```python
from build123d import *

# Parameters (mm, degrees)
BOSS_EXTRUDE2_START      = 6
BOSS_EXTRUDE2_DEPTH      = 44
SKETCH2_R                = 16.25
CUT_EXTRUDE1_DEPTH       = 1
CUT_EXTRUDE1_DEPTH_BACK  = 45
CUT_EXTRUDE3_DEPTH       = 45
FILLET1_R                = 3
SKETCH5_W                = 35
SKETCH5_H                = 25
CUT_EXTRUDE4_DEPTH       = 10
FILLET2_R                = 3
SKETCH6_R                = 16.25
SKETCH6_R_2              = 9.5
SKETCH6_R_3              = 1.65
BOSS_EXTRUDE3_DEPTH      = 5
SKETCH7_R                = 2.25
CUT_EXTRUDE5_DEPTH       = 26
CUT_EXTRUDE5_DEPTH_BACK  = 26
CUT_EXTRUDE6_REACH       = 60.55
SKETCH8_R                = 1.175
BOSS_EXTRUDE4_START      = -44
BOSS_EXTRUDE4_DEPTH      = 8
BOSS_EXTRUDE4_DEPTH_BACK = 10
FILLET5_R                = 0.25
FILLET6_R                = 0.25


with BuildPart() as part:
    # Sketch1 → Boss-Extrude2 (new body)
    with BuildSketch(Plane.XY.offset(BOSS_EXTRUDE2_START)):
        with BuildLine():
            Line((-25, 0), (-25, -29.344548046))
            Line((-25, -29.344548046), (-25, -32.344548046))
            Line((-25, -32.344548046), (-20.974572981, -32.344548046))
            Line((-20.974572981, -32.344548046), (-20.974572981, -35.344548046))
            Line((-20.974572981, -35.344548046), (-15.390432855, -35.344548046))
            ThreePointArc((-15.390432855, -35.344548046), (0, -38.55), (15.390432855, -35.344548046))
            Line((15.390432855, -35.344548046), (20.974572981, -35.344548046))
            Line((20.974572981, -35.344548046), (20.974572981, -32.344548046))
            Line((20.974572981, -32.344548046), (25, -32.344548046))
            Line((25, -32.344548046), (25, -29.344548046))
            Line((25, -29.344548046), (25, 0))
            Line((25, 0), (25, 20))
            Line((25, 20), (-25, 20))
            Line((-25, 20), (-25, 0))
        make_face()
    extrude(amount=BOSS_EXTRUDE2_DEPTH)

    # Sketch2 → Cut-Extrude1 (cut, two sides)
    with BuildSketch(Plane.XY.offset(50)) as cut_extrude1_sk:
        with Locations((0, -10)):
            Circle(SKETCH2_R)
    extrude(amount=CUT_EXTRUDE1_DEPTH, mode=Mode.SUBTRACT)
    extrude(cut_extrude1_sk.sketch, amount=-CUT_EXTRUDE1_DEPTH_BACK, mode=Mode.SUBTRACT)

    # Sketch4 → Cut-Extrude3 (cut, through all)
    with BuildSketch(Plane.XY.offset(50)):
        with BuildLine():
            Line((-23, 18), (23, 18))
            Line((23, 18), (23, 2))
            Line((23, 2), (14.317821063, 2))
            ThreePointArc((14.317821063, 2), (0, 8.681541692), (-14.317821063, 2))
            Line((-14.317821063, 2), (-23, 2))
            Line((-23, 2), (-23, 18))
        make_face()
    extrude(amount=-CUT_EXTRUDE3_DEPTH, mode=Mode.SUBTRACT)

    # Fillet1
    fillet1_edges = [part.edges().sort_by_distance(p)[0] for p in [
        (23, 18, 28),
        (23, 2, 28),
        (14.317821063, 2, 28),
        (-14.317821063, 2, 28),
        (-23, 2, 28),
        (-23, 18, 28),
    ]]
    fillet(fillet1_edges, radius=FILLET1_R)

    # Sketch5 → Cut-Extrude4 (cut)
    with BuildSketch(Plane(origin=(0, 20, 0), x_dir=(1, 0, 0), z_dir=(0, 1, 0))):
        with Locations((0, -37.5)):
            Rectangle(SKETCH5_W, SKETCH5_H)
    extrude(amount=-CUT_EXTRUDE4_DEPTH, mode=Mode.SUBTRACT)

    # Fillet2
    fillet2_edges = [part.edges().sort_by_distance(p)[0] for p in [
        (17.5, 19, 50),
        (17.5, 19, 25),
        (-17.5, 19, 25),
        (-17.5, 19, 50),
    ]]
    fillet(fillet2_edges, radius=FILLET2_R)

    # Sketch6 → Boss-Extrude3 (add)
    with BuildSketch(Plane.XY.offset(14)):
        with Locations((0, -10)):
            Circle(SKETCH6_R)
        with Locations((0, -10)):
            Circle(SKETCH6_R_2, mode=Mode.SUBTRACT)
        with Locations((4.446261863, 2.21600407)):
            Circle(SKETCH6_R_3, mode=Mode.SUBTRACT)
        with Locations((12.21600407, -14.446261863)):
            Circle(SKETCH6_R_3, mode=Mode.SUBTRACT)
        with Locations((-4.446261863, -22.21600407)):
            Circle(SKETCH6_R_3, mode=Mode.SUBTRACT)
        with Locations((-12.21600407, -5.553738137)):
            Circle(SKETCH6_R_3, mode=Mode.SUBTRACT)
    extrude(amount=-BOSS_EXTRUDE3_DEPTH)

    # Sketch7 → Cut-Extrude5 (cut, two sides)
    with BuildSketch(Plane(origin=(0, 0, 0), x_dir=(0, 0, -1), z_dir=(1, 0, 0))) as cut_extrude5_sk:
        with Locations((-40.3, -32)):
            Circle(SKETCH7_R)
        with Locations((-10.3, -32)):
            Circle(SKETCH7_R)
    extrude(amount=CUT_EXTRUDE5_DEPTH, mode=Mode.SUBTRACT)
    extrude(cut_extrude5_sk.sketch, amount=-CUT_EXTRUDE5_DEPTH_BACK, mode=Mode.SUBTRACT)

    # Sketch8 → Cut-Extrude6 (cut, up to next)
    with BuildSketch(Plane(origin=(0, 20, 0), x_dir=(1, 0, 0), z_dir=(0, 1, 0)), mode=Mode.PRIVATE) as cut_extrude6_sk1:
        with Locations((-4.75, -16.8)):
            Circle(SKETCH8_R)
    cut_extrude6_tool1 = extrude(cut_extrude6_sk1.sketch, amount=-CUT_EXTRUDE6_REACH, mode=Mode.PRIVATE) & part.part
    add(cut_extrude6_tool1.solids().sort_by_distance((-4.75, 20, 16.8))[0], mode=Mode.SUBTRACT)
    # Sketch8 → Cut-Extrude6 (cut, up to next)
    with BuildSketch(Plane(origin=(0, 20, 0), x_dir=(1, 0, 0), z_dir=(0, 1, 0)), mode=Mode.PRIVATE) as cut_extrude6_sk2:
        with Locations((4.75, -16.8)):
            Circle(SKETCH8_R)
    cut_extrude6_tool2 = extrude(cut_extrude6_sk2.sketch, amount=-CUT_EXTRUDE6_REACH, mode=Mode.PRIVATE) & part.part
    add(cut_extrude6_tool2.solids().sort_by_distance((4.75, 20, 16.8))[0], mode=Mode.SUBTRACT)

    # Sketch9 → Boss-Extrude4 (add, two sides)
    with BuildSketch(Plane.XY.offset(50).offset(BOSS_EXTRUDE4_START)) as boss_extrude4_sk:
        with BuildLine():
            ThreePointArc((-14.655326574, 2.171572875), (-15.148020638, 2.043204321), (-15.655326574, 2))
            Line((-15.655326574, 2), (-15.655326574, 1))
            ThreePointArc((-15.655326574, 1), (-14.085187018, 1.32105154), (-12.767095323, 2.232669113))
            ThreePointArc((-12.767095323, 2.232669113), (0, 7.681541692), (12.767095323, 2.232669113))
            ThreePointArc((12.767095323, 2.232669113), (14.085187018, 1.32105154), (15.655326574, 1))
            Line((15.655326574, 1), (15.655326574, 2))
            ThreePointArc((15.655326574, 2), (15.148020638, 2.043204321), (14.655326574, 2.171572875))
            ThreePointArc((14.655326574, 2.171572875), (14.028093012, 2.479660552), (13.489153136, 2.924501835))
            ThreePointArc((13.489153136, 2.924501835), (0, 8.681541692), (-13.489153136, 2.924501835))
            ThreePointArc((-13.489153136, 2.924501835), (-14.028093012, 2.479660552), (-14.655326574, 2.171572875))
        make_face()
        with BuildLine():
            Line((-15.655326574, 11.412284527), (-15.655326574, 2))
            ThreePointArc((-15.655326574, 2), (-15.148020638, 2.043204321), (-14.655326574, 2.171572875))
            Line((-14.655326574, 2.171572875), (-14.655326574, 10.53248927))
            ThreePointArc((-14.655326574, 10.53248927), (-14.566443026, 10.944638287), (-14.31559295, 11.283520769))
            ThreePointArc((-14.31559295, 11.283520769), (0, 16.681541692), (14.31559295, 11.283520769))
            ThreePointArc((14.31559295, 11.283520769), (14.566443026, 10.944638287), (14.655326574, 10.53248927))
            Line((14.655326574, 10.53248927), (14.655326574, 2.171572875))
            ThreePointArc((14.655326574, 2.171572875), (15.148020638, 2.043204321), (15.655326574, 2))
            Line((15.655326574, 2), (15.655326574, 11.412284527))
            ThreePointArc((15.655326574, 11.412284527), (0, 17.681541692), (-15.655326574, 11.412284527))
        make_face()
    extrude(amount=BOSS_EXTRUDE4_DEPTH)
    extrude(boss_extrude4_sk.sketch, amount=-BOSS_EXTRUDE4_DEPTH_BACK)

    # Fillet5
    fillet5_edges = [part.edges().sort_by_distance(p)[0] for p in [
        (0, 8.681541692, -4),
        (14.566443026, 10.944638287, -4),
        (0, 16.681541692, -4),
        (-14.566443026, 10.944638287, -4),
        (-14.028093012, 2.479660552, -4),
        (14.028093012, 2.479660552, -4),
        (14.655326574, 6.352031072, -4),
        (-14.655326574, 6.352031072, -4),
    ]]
    fillet(fillet5_edges, radius=FILLET5_R)

    # Fillet6
    fillet6_edges = [part.edges().sort_by_distance(p)[0] for p in [
        (-14.655326574, 6.352031072, 14),
        (0, 16.681541692, 14),
        (14.566443026, 10.944638287, 14),
        (14.655326574, 6.352031072, 14),
        (-14.566443026, 10.944638287, 14),
    ]]
    fillet(fillet6_edges, radius=FILLET6_R)


solid = part.part
```
The model under review builds one solid part; all positions refer to its coordinate system, in mm. A direction names the side the tool comes from. Round coordinates to 2 decimals unless told otherwise and drop trailing zeros. Loops run counter-clockwise (first coordinate to the right, second up) from the corner with the lowest first, then second, coordinate; pieces in that order, holes last.
1) The part is to be moulded in two halves that separate along X. For faces 6 (the face through (23, -32.345, 25)), 7 (the face through (15.5, -5.12, 7.52)), say which applies: pulls with the +X half, pulls with the -X half, needs draft (parallel to the pull), parting line crosses it, or undercut.
Values follow:
face 6: needs draft
face 7: undercut
2) Consider section B-B on z = 40.3. State the section outline as (x, y) points.
Values follow:
outline: (-25, -29.75) - (25, -29.75) - (25, 20) - (17.5, 20) - (17.5, 18) - (20, 18) arc R3 cw to (23, 15) - (23, 5) arc R3 cw to (20, 2) - (15.66, 2) arc R3 cw to (13.49, 2.92) arc R18.68 ccw to (-13.49, 2.92) arc R3 cw to (-15.66, 2) - (-20, 2) arc R3 cw to (-23, 5) - (-23, 15) arc R3 cw to (-20, 18) - (-17.5, 18) - (-17.5, 20) - (-25, 20) - close; (-20.97, -35.34) - (-15.39, -35.34) arc R38.55 ccw to (15.39, -35.34) - (20.97, -35.34) - (20.97, -34.25) - (-20.97, -34.25) - close; hole circle Ø32.5 at (0, -10)
3) Consider section D-D on x = 0. Give the number of separate pieces and of enclosed holes in the cut face, then the cut area to 3 significant figures.
Values follow:
separate pieces: 4
enclosed holes: 2
area: 750 mm2
4) Wall thickness on line 1 along X through (y, z) = (-17, 20.5) (3 decimals); line 2 along X through (y, z) = (-7, 13); line 3 along X through (y, z) = (4.5, 32): over which ranges is each line inside the solid? List them lowest first.
Values follow:
line 1: x = -25 to -14.665, 14.665 to 25
line 2: x = -25 to -13.01, -11.42 to -9.01, 9.01 to 25
line 3: x = -25 to -22.96, -11.78 to -7.34, 7.34 to 11.78, 22.96 to 25
5) Consider section C-C on z = 1. State the section outline as (x, y) points, then the cut area to 3 significant figures.
Values follow:
outline: (-15.66, 1) arc R4 ccw to (-12.77, 2.23) arc R17.68 cw to (12.77, 2.23) arc R4 ccw to (15.66, 1) - (15.66, 11.41) arc R22.68 ccw to (-15.66, 11.41) - close; hole (-14.66, 2.17) arc R3 ccw to (-13.49, 2.92) arc R18.68 cw to (13.49, 2.92) arc R3 ccw to (14.66, 2.17) - (14.66, 10.53) arc R1 ccw to (14.32, 11.28) arc R21.68 ccw to (-14.32, 11.28) arc R1 ccw to (-14.66, 10.53) - close
area: 86.7 mm2
6) Consider section A-A on y = -10. State the section outline as (x, z) points.
Values follow:
outline: (-25, 6) - (-16.25, 6) - (-16.25, 9) - (-9.5, 9) - (-9.5, 14) - (-16.25, 14) - (-16.25, 50) - (-25, 50) - close; (9.5, 9) - (16.25, 9) - (16.25, 6) - (25, 6) - (25, 50) - (16.25, 50) - (16.25, 14) - (9.5, 14) - close
7) Tool access review of faces 1 (the face through (15.5, -5.12, 32.25)), 2 (the face through (18, -35.345, 28)), 3 (the face through (18, 2, 28)), 4 (the face through (14.06, 1.33, 1.07)), 5 (the face through (-17.5, 19, 38)): name each direction out of +Z, -Z, +X, -X, +Y, -Y from which nothing blocks a thin tool from reaching the whole face with its end or side.
Values follow:
face 1: +Z
face 2: +Z, -Z, +X, -Y
face 3: +Z, -Z
face 4: -Z, -Y
face 5: +Z, +Y
8) Clearance check with flat-ended pins moving along their axes: P1, Ø10, axis at x = 2, y = -8.5, coming from the -Z side; P2, Ø8, axis at x = 15.5, z = 7, coming from the -Y side; P3, Ø1.5, axis at y = -34, z = 32.5, coming from the -X side; P4, Ø4, axis at x = -12.22, y = -5.55, coming from the -Z side. State where each tip first meets the part, or that it passes through.
Values follow:
P1: passes through
P2: stops at y = -36.79
P3: stops at x = -20.97
P4: stops at z = 9
